Work out the finished part from the listing and answer in its coordinate system (mm). Face numbers are marked on the shaded views. A direction names the side the tool comes from. Give positions to 0.01 mm unless a question says otherwise; leave off trailing zeros. Loops run counter-clockwise (first coordinate to the right, second up) from the corner with the lowest first, then second, coordinate; pieces in that order, holes last. Notation, with made-up numbers: M 80,-4 L 104,-4 A12 ccw 104,17 Z; hole C 87.5,81.5 d1. An arc over 180 degrees is marked long. Use a Markdown table: item, result.
```python
from build123d import *

# Parameters (mm, degrees)
F1_DEPTH = 57
F3_DEPTH = 40


# Not quite as in the source:
# - a feature of the source that left no trace in its solid (it failed there, or was rolled back) is left out


with BuildPart() as f1:
    # F0 (on Front) → F1 (new body)
    with BuildSketch(Plane.XZ):
        with BuildLine():
            ThreePointArc((-15.6, 0), (-11.0308657865, 11.0308657865), (0, 15.6))
            Line((0, 15.6), (-40, 15.6))
            Line((-40, 15.6), (-40, 0))
            Line((-40, 0), (-15.6, 0))
        make_face()
        with BuildLine():
            ThreePointArc((10.5734336902, -0.75), (-10.6, 0), (10.5734336902, 0.75))
            Line((10.5734336902, 0.75), (15.5819607239, 0.75))
            ThreePointArc((15.5819607239, 0.75), (15.2481384312, 3.2945825812), (14.5016378385, 5.75))
            ThreePointArc((14.5016378385, 5.75), (8.765272386, 12.9046503246), (0, 15.6))
            ThreePointArc((0, 15.6), (-11.0308657865, 11.0308657865), (-15.6, 0))
            ThreePointArc((-15.6, 0), (-2.9269822103, -15.3229492964), (14.5016378385, -5.75))
            ThreePointArc((14.5016378385, -5.75), (15.2481384312, -3.2945825812), (15.5819607239, -0.75))
            Line((15.5819607239, -0.75), (10.5734336902, -0.75))
        make_face()
        with BuildLine():
            ThreePointArc((14.5016378385, 5.75), (15.2481384312, 3.2945825812), (15.5819607239, 0.75))
            Line((15.5819607239, 0.75), (22.5016378385, 0.75))
            Line((22.5016378385, 0.75), (22.5016378385, 5.75))
            Line((22.5016378385, 5.75), (14.5016378385, 5.75))
        make_face()
        with BuildLine():
            Line((22.5016378385, -0.75), (15.5819607239, -0.75))
            ThreePointArc((15.5819607239, -0.75), (15.2481384312, -3.2945825812), (14.5016378385, -5.75))
            Line((14.5016378385, -5.75), (22.5016378385, -5.75))
            Line((22.5016378385, -5.75), (22.5016378385, -0.75))
        make_face()
    extrude(amount=F1_DEPTH)

    # F2 (on face) → F3 (join)
    with BuildSketch(Plane(origin=(-40, 0, 0), x_dir=(0, -1, 0), z_dir=(-1, 0, 0))):
        Polygon((25.45, 17.055), (24, 15.6), (33, 15.6), (31.55, 17.055), align=None)
    extrude(amount=-F3_DEPTH)


solid = f1.part
```
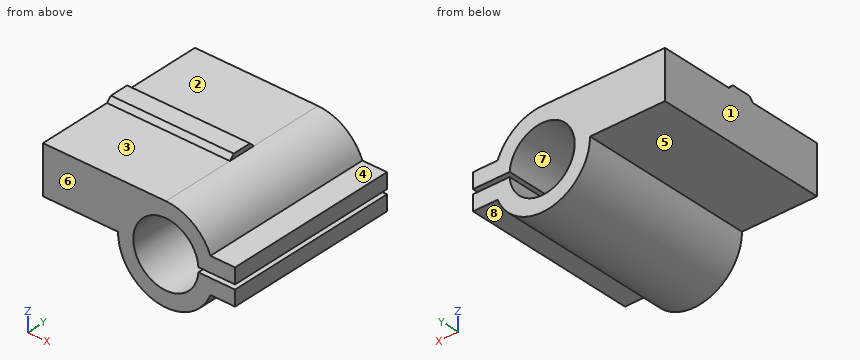
(1) The mould has two halves that part along Z. Classify the marked faces 6, 7 and 8: released by +Z, released by -Z, zero draft, split by the parting line, or undercut.
Entries:
| item | result |
|---|---|
| face 6 | zero draft |
| face 7 | undercut |
| face 8 | released by -Z |
(2) Which of the six approach directions +Z, -Z, +X, -X, +Y, -Y give full straight-line access (tool end or side, diameter ignored) to the marked faces 1, 2, 3, 4 and 5?
Entries:
| item | result |
|---|---|
| face 1 | +Z, -Z, -X, +Y, -Y |
| face 2 | +Z, +X, -X, +Y |
| face 3 | +Z, +X, -X, -Y |
| face 4 | +Z, +X, +Y, -Y |
| face 5 | -Z, -X, +Y, -Y |
(3) A cutting plane is placed at D-D (x = -36). Write down the section's boundary in (y, z) (3 decimals), and give its area (3 significant figures).
Entries:
| item | result |
|---|---|
| outline | M -57,0 L 0,0 L 0,15.6 L -24,15.6 L -25.45,17.055 L -31.55,17.055 L -33,15.6 L -57,15.6 Z |
| area | 900 mm² |
(4) A cutting plane is placed at A-A (x = 3). Write down the section's boundary in (y, z).
Entries:
| item | result |
|---|---|
| outline | M -57,-15.31 L 0,-15.31 L 0,-10.17 L -57,-10.17 Z; M -57,10.17 L 0,10.17 L 0,15.31 L -57,15.31 Z |
(5) Consider probe 1 along Z at (x, y) = (0, -17); probe 2 along X at (y, z) = (-15, -0.5); probe 3 along X at (y, z) = (-30, 2.5). Determine where each line is inside the solid, lowest interval first. Write a range as [from, to].
Entries:
| item | result |
|---|---|
| probe 1 | z = [-15.6, -10.6], [10.6, 15.6] |
| probe 2 | x = [-15.59, -10.59] |
| probe 3 | x = [-40, -10.3], [10.3, 22.5] |
(6) A cutting plane is placed at B-B (z = 6.5). Write down the section's boundary in (x, y), and give its area (3 significant figures).
Entries:
| item | result |
|---|---|
| outline | M -40,-57 L -8.37,-57 L -8.37,0 L -40,0 Z; M 8.37,-57 L 14.18,-57 L 14.18,0 L 8.37,0 Z |
| area | 2,130 mm² |
(7) A cutting plane is placed at C-C (y = -17.5). Write down the section's boundary in (x, z).
Entries:
| item | result |
|---|---|
| outline | M -40,0 L -15.6,0 A15.6 ccw 14.5,-5.75 L 22.5,-5.75 L 22.5,-0.75 L 10.57,-0.75 A10.6 cw long 10.57,0.75 L 22.5,0.75 L 22.5,5.75 L 14.5,5.75 A15.6 ccw 0,15.6 L -40,15.6 Z |
(8) Given P1, Ø9.5, axis at x = 18.5, y = -24.5, coming from the -Z side; P2, Ø6, axis at x = 15.5, y = -22.5, coming from the +Z side; P3, Ø2, axis at x = -29.5, y = -10, coming from the -Z side, each flat-ended and moving along its own axis, determine where each tip first touches the part or whether it passes through.
Entries:
| item | result |
|---|---|
| P1 | stops at z = -7.37 |
| P2 | stops at z = 9.33 |
| P3 | stops at z = 0 |
